Here's how the part is built. I have some questions about the finished solid (model axes, mm). Coordinates: 2 decimals unless noted, no trailing zeros. Write each loop counter-clockwise with the first axis right and the second up, starting at its lowest first coordinate (ties: lowest second). Pieces come first, ordered by that corner, then holes. Notation, with made-up numbers: M 76.25,6 L 120.25,6 A29 ccw 120.25,44 Z; hole C 76,53 d6. An arc over 180 degrees is marked long. Use a Markdown table: item, result.
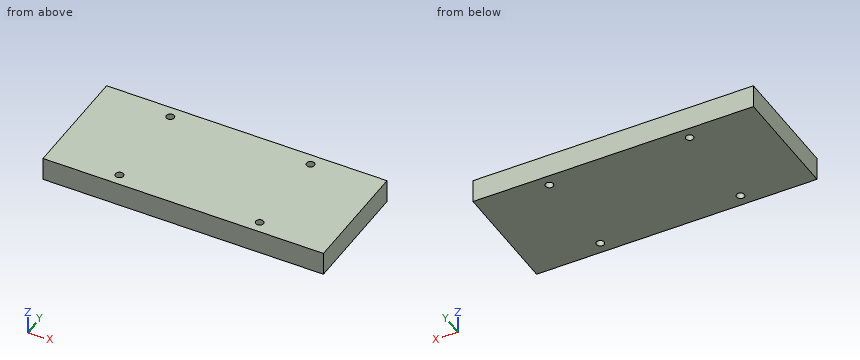
```python
from build123d import *

# Parameters (mm, degrees)
F0_W       = 457.2
F0_H       = 38.1
F1_DEPTH   = 95.25
F4_D       = 12.7
F4_DEPTH   = 609.6
F4_TIP     = 3.8154649308
F4_2_D     = 12.7
F4_2_DEPTH = 609.6
F4_2_TIP   = 3.8154649308
F5_D       = 12.7
F5_DEPTH   = 609.6
F5_TIP     = 3.8154649308
F5_2_D     = 12.7
F5_2_DEPTH = 609.6
F5_2_TIP   = 3.8154649308
F6_D       = 12.7
F6_DEPTH   = 609.6
F6_TIP     = 3.8154649308
F6_2_D     = 12.7
F6_2_DEPTH = 609.6
F6_2_TIP   = 3.8154649308
F7_D       = 12.7
F7_DEPTH   = 609.6
F7_TIP     = 3.8154649308
F7_2_D     = 12.7
F7_2_DEPTH = 609.6
F7_2_TIP   = 3.8154649308


# Not quite as in the source:
# - a feature names something its author has since deleted; it is built from what else it names


with BuildPart() as f1:
    # F0 (on Front) → F1 (new body, symmetric)
    with BuildSketch(Plane.XZ):
        Rectangle(F0_W, F0_H)
    extrude(amount=F1_DEPTH, both=True)


with BuildPart() as f2_1:
    # F2: copy of F1
    add(f1.part.moved(Location((0, 0, 152.4))))

    # F4#2
    with Locations(Plane.XY.offset(171.45)):
        with Locations((-114.3, 76.2)):
            Hole(F4_2_D / 2, depth=F4_2_DEPTH)
            with Locations((0, 0, -(F4_2_DEPTH + F4_2_TIP / 2))):  # 118° drill point
                Cone(0, F4_2_D / 2, F4_2_TIP, mode=Mode.SUBTRACT)

    # F5#2
    with Locations(Plane.XY.offset(171.45)):
        with Locations((114.3, 76.2)):
            Hole(F5_2_D / 2, depth=F5_2_DEPTH)
            with Locations((0, 0, -(F5_2_DEPTH + F5_2_TIP / 2))):  # 118° drill point
                Cone(0, F5_2_D / 2, F5_2_TIP, mode=Mode.SUBTRACT)

    # F6#2
    with Locations(Plane.XY.offset(171.45)):
        with Locations((-114.3, -76.2)):
            Hole(F6_2_D / 2, depth=F6_2_DEPTH)
            with Locations((0, 0, -(F6_2_DEPTH + F6_2_TIP / 2))):  # 118° drill point
                Cone(0, F6_2_D / 2, F6_2_TIP, mode=Mode.SUBTRACT)

    # F7#2
    with Locations(Plane.XY.offset(171.45)):
        with Locations((114.3, -76.2)):
            Hole(F7_2_D / 2, depth=F7_2_DEPTH)
            with Locations((0, 0, -(F7_2_DEPTH + F7_2_TIP / 2))):  # 118° drill point
                Cone(0, F7_2_D / 2, F7_2_TIP, mode=Mode.SUBTRACT)


with BuildPart() as f1_1:
    add(f1.part)

    # F4
    with Locations(Plane.XY.offset(171.45)):
        with Locations((-114.3, 76.2)):
            Hole(F4_D / 2, depth=F4_DEPTH)
            with Locations((0, 0, -(F4_DEPTH + F4_TIP / 2))):  # 118° drill point
                Cone(0, F4_D / 2, F4_TIP, mode=Mode.SUBTRACT)

    # F5
    with Locations(Plane.XY.offset(171.45)):
        with Locations((114.3, 76.2)):
            Hole(F5_D / 2, depth=F5_DEPTH)
            with Locations((0, 0, -(F5_DEPTH + F5_TIP / 2))):  # 118° drill point
                Cone(0, F5_D / 2, F5_TIP, mode=Mode.SUBTRACT)

    # F6
    with Locations(Plane.XY.offset(171.45)):
        with Locations((-114.3, -76.2)):
            Hole(F6_D / 2, depth=F6_DEPTH)
            with Locations((0, 0, -(F6_DEPTH + F6_TIP / 2))):  # 118° drill point
                Cone(0, F6_D / 2, F6_TIP, mode=Mode.SUBTRACT)

    # F7
    with Locations(Plane.XY.offset(171.45)):
        with Locations((114.3, -76.2)):
            Hole(F7_D / 2, depth=F7_DEPTH)
            with Locations((0, 0, -(F7_DEPTH + F7_TIP / 2))):  # 118° drill point
                Cone(0, F7_D / 2, F7_TIP, mode=Mode.SUBTRACT)


solid = f1_1.part
```
1. I need wall thicknesses on probe 1 along X at (y, z) = (76, 6); probe 2 along Y at (x, z) = (-114, -5). Which ranges of each line are inside material? Lowest first, please.
Answers follow:
| item | result |
|---|---|
| probe 1 | x = -228.6 to -120.65, -107.95 to 107.95, 120.65 to 228.6 |
| probe 2 | y = -95.25 to -82.54, -69.86 to 69.86, 82.54 to 95.25 |
2. Suppose I cut it at A-A on y = 76.2. Write out the boundary of the cut face in (x, z).
Answers follow:
| item | result |
|---|---|
| outline | M -228.6,-19.05 L -120.65,-19.05 L -120.65,19.05 L -228.6,19.05 Z; M -107.95,-19.05 L 107.95,-19.05 L 107.95,19.05 L -107.95,19.05 Z; M 120.65,-19.05 L 228.6,-19.05 L 228.6,19.05 L 120.65,19.05 Z |
3. Suppose I cut it at B-B on x = -114.3. Write out the boundary of the cut face in (y, z), and give its area (3 significant figures).
Answers follow:
| item | result |
|---|---|
| outline | M -95.25,-19.05 L -82.55,-19.05 L -82.55,19.05 L -95.25,19.05 Z; M -69.85,-19.05 L 69.85,-19.05 L 69.85,19.05 L -69.85,19.05 Z; M 82.55,-19.05 L 95.25,-19.05 L 95.25,19.05 L 82.55,19.05 Z |
| area | 6,290 mm2 |
4. Will this pin go through, and if not, where does the flat tip stop? pin 1 Ø7.5 at (x, y) = (-114.3, -76.2) entering from -Z.
Answers follow:
| item | result |
|---|---|
| pin 1 | passes through |
